Part print with two shaded views. Sizes in mm from the minimum x, y, z corner. A direction names the side the tool comes from. Round coordinates to 2 decimals unless told otherwise and drop trailing zeros. Loops run counter-clockwise (first coordinate to the right, second up) from the corner with the lowest first, then second, coordinate; pieces in that order, holes last.
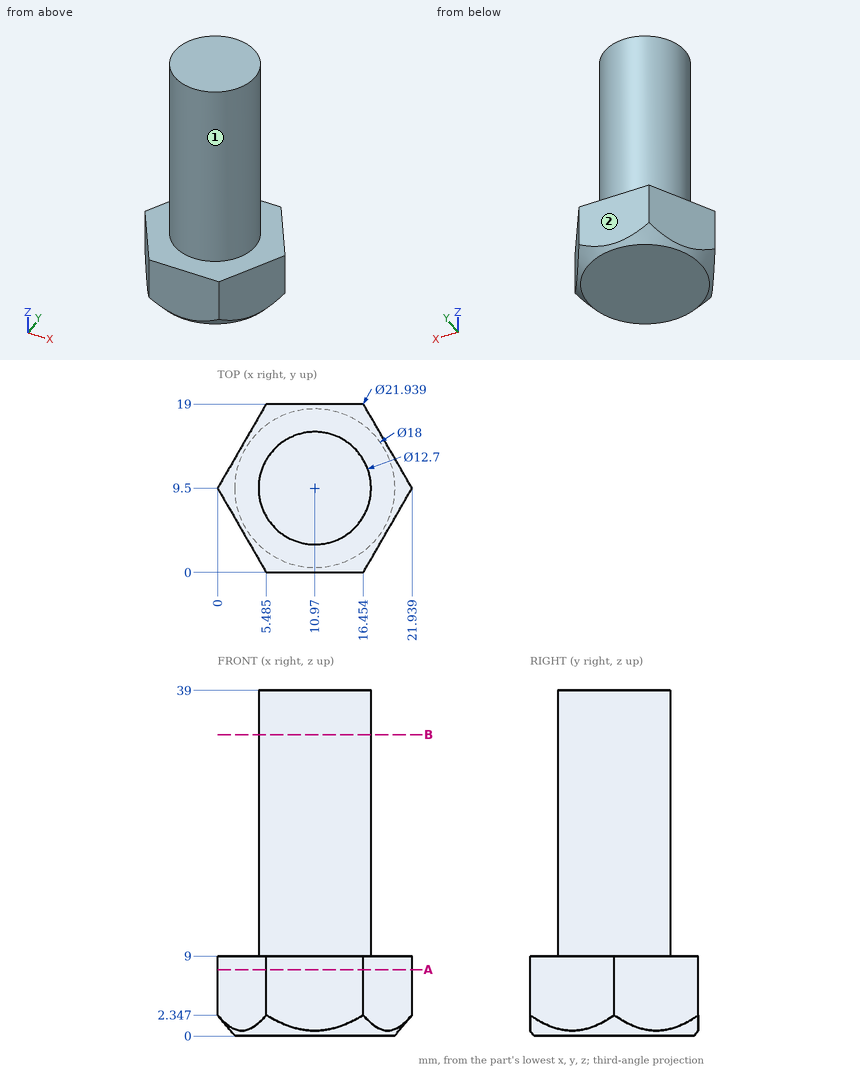
Item 1: Cut at A-A (z = 7.5). List the corners of the cut face in (x, y) (1 decimal), plus the area to 3 significant figures.
Verdict:
outline: (0, 9.5) - (5.5, 0) - (16.5, 0) - (21.9, 9.5) - (16.5, 19) - (5.5, 19) - close
area: 313 mm2
Item 2: 3-axis set-ups, long thin cutter, end or side, ignore diameter. For the marked faces 1 and 2: which of +Z, -Z, +X, -X, +Y, -Y reach the whole face in a straight line?
Verdict:
face 1: +Z
face 2: +Z, -Z, +X, -X, +Y
Item 3: Flat gauge pins, fed straight in: P1, Ø1.5, axis at x = 15, y = 4, coming from the +Z side; P2, Ø1.5, axis at y = 14, z = 26, coming from the -X side (1 decimal); P3, Ø1, axis at x = 8.5, z = 13, coming from the +Y side; P4, Ø4, axis at y = 6.5, z = 6, coming from the +X side. Where does each tip first touch, or does it go through?
Verdict:
P1: stops at z = 39
P2: stops at x = 5.8
P3: stops at y = 15.54
P4: stops at x = 21.36
Item 4: Cut at B-B (z = 34). List the corners of the cut face in (x, y), plus the area to 3 significant figures.
Verdict:
outline: circle Ø12.7 at (10.97, 9.5)
area: 127 mm2
Item 5: Wall check: L1, parallel to X at y = 9.75, z = 30.5 (1 decimal); L2, parallel to Y at x = 10.75, z = 26; L3, parallel to Z at x = 17.5, y = 11. Give the ranges that are in metal, low to high.
Verdict:
L1: x = 4.6 to 17.3
L2: y = 3.15 to 15.85
L3: z = 0 to 9
